```python
from build123d import *

# Parameters (mm, degrees)
ESTRUSIONE_ESTRUSIONE1_DEPTH      = 48
ESTRUSIONE_ESTRUSIONE1_DEPTH_BACK = 5
SCHIZZO2_W                        = 45
SCHIZZO2_H                        = 3
ESTRUSIONE_ESTRUSIONE2_DEPTH      = 5
CORPO_SPOSTA_COPIA1_START         = 131.104025403
CORPO_SPOSTA_COPIA1_OUTLINE_W     = 3
CORPO_SPOSTA_COPIA1_OUTLINE_H     = 43
CORPO_SPOSTA_COPIA1_DEPTH         = 31.786555516
CORPO_SPOSTA_COPIA1_2_OUTLINE_W   = 3
CORPO_SPOSTA_COPIA1_2_OUTLINE_H   = 5
CORPO_SPOSTA_COPIA1_2_DEPTH       = 5
CORPO_SPOSTA_COPIA1_START_2       = 157.890580919
CORPO_SPOSTA_COPIA1_3_OUTLINE_W   = 3
CORPO_SPOSTA_COPIA1_3_OUTLINE_H   = 5
CORPO_SPOSTA_COPIA1_3_DEPTH       = 5
CORPO_SPOSTA_COPIA1_4_OUTLINE_W   = 3
CORPO_SPOSTA_COPIA1_4_OUTLINE_H   = 45
CORPO_SPOSTA_COPIA1_4_DEPTH       = 31.786555516
CORPO_SPOSTA_COPIA1_START_3       = 136.104025403
CORPO_SPOSTA_COPIA1_5_OUTLINE_W   = 3
CORPO_SPOSTA_COPIA1_5_OUTLINE_H   = 3
CORPO_SPOSTA_COPIA1_5_DEPTH       = 21.786555516


# Read off the part's stored shape, not the designer's step: Corpo-Sposta/copia1
with BuildPart() as part:
    # Schizzo1 → Estrusione-Estrusione1 (new, two sides: drawn at the far end of the back side and taken through both)
    with BuildSketch(Plane.XY.offset(-ESTRUSIONE_ESTRUSIONE1_DEPTH_BACK)):
        Polygon((198.017140331, -69.250735791), (177.803209237, -77.377911869), (178.92231814, -80.161362114), (199.136249234, -72.034186035), align=None)
    extrude(amount=ESTRUSIONE_ESTRUSIONE1_DEPTH + ESTRUSIONE_ESTRUSIONE1_DEPTH_BACK)

    # Schizzo2 → Estrusione-Estrusione2 (add)
    with BuildSketch(Plane(origin=(146.49352536, 58.898918246, 0), x_dir=(0, 0, -1), z_dir=(0.9278167482016688, 0.3730363008562049, 0))):
        with Locations((-22.5, -139.619574027)):
            Rectangle(SCHIZZO2_W, SCHIZZO2_H)
    estrusione_estrusione2 = extrude(amount=ESTRUSIONE_ESTRUSIONE2_DEPTH)

    # Specchia1: Estrusione-Estrusione2 across plane
    add(estrusione_estrusione2.mirror(Plane(origin=(136.386559813, 54.835330207, 0), x_dir=(0, 0, 1), z_dir=(0.9278167482016688, 0.37303630085620504, 0))))

    # Corpo-Sposta/copia1 outline → Corpo-Sposta/copia1 (cut)
    with BuildSketch(Plane(origin=(0, 0, 0), x_dir=(-0.373036300856202, 0.92781674820167, 0), z_dir=(0.92781674820167, 0.373036300856202, 0)).offset(CORPO_SPOSTA_COPIA1_START)):
        with Locations((-139.619574027, 26.5)):
            Rectangle(CORPO_SPOSTA_COPIA1_OUTLINE_W, CORPO_SPOSTA_COPIA1_OUTLINE_H)
    extrude(amount=CORPO_SPOSTA_COPIA1_DEPTH, mode=Mode.SUBTRACT)

    # Corpo-Sposta_copia1 2 outline → Corpo-Sposta_copia1 2 (cut)
    with BuildSketch(Plane(origin=(0, 0, 0), x_dir=(-0.373036300856202, 0.92781674820167, 0), z_dir=(0.92781674820167, 0.373036300856202, 0)).offset(CORPO_SPOSTA_COPIA1_START)):
        with Locations((-139.619574027, 2.5)):
            Rectangle(CORPO_SPOSTA_COPIA1_2_OUTLINE_W, CORPO_SPOSTA_COPIA1_2_OUTLINE_H)
    extrude(amount=CORPO_SPOSTA_COPIA1_2_DEPTH, mode=Mode.SUBTRACT)

    # Corpo-Sposta_copia1 3 outline → Corpo-Sposta_copia1 3 (cut)
    with BuildSketch(Plane(origin=(0, 0, 0), x_dir=(-0.373036300856202, 0.92781674820167, 0), z_dir=(0.92781674820167, 0.373036300856202, 0)).offset(CORPO_SPOSTA_COPIA1_START_2)):
        with Locations((-139.619574027, 2.5)):
            Rectangle(CORPO_SPOSTA_COPIA1_3_OUTLINE_W, CORPO_SPOSTA_COPIA1_3_OUTLINE_H)
    extrude(amount=CORPO_SPOSTA_COPIA1_3_DEPTH, mode=Mode.SUBTRACT)

    # Corpo-Sposta_copia1 4 outline → Corpo-Sposta_copia1 4 (add)
    with BuildSketch(Plane(origin=(0, 0, 0), x_dir=(-0.373036300856202, 0.92781674820167, 0), z_dir=(0.92781674820167, 0.373036300856202, 0)).offset(CORPO_SPOSTA_COPIA1_START)):
        with Locations((-139.619574027, -22.5)):
            Rectangle(CORPO_SPOSTA_COPIA1_4_OUTLINE_W, CORPO_SPOSTA_COPIA1_4_OUTLINE_H)
    extrude(amount=CORPO_SPOSTA_COPIA1_4_DEPTH)

    # Corpo-Sposta_copia1 5 outline → Corpo-Sposta_copia1 5 (add)
    with BuildSketch(Plane(origin=(0, 0, 0), x_dir=(-0.373036300856202, 0.92781674820167, 0), z_dir=(0.92781674820167, 0.373036300856202, 0)).offset(CORPO_SPOSTA_COPIA1_START_3)):
        with Locations((-139.619574027, -46.5)):
            Rectangle(CORPO_SPOSTA_COPIA1_5_OUTLINE_W, CORPO_SPOSTA_COPIA1_5_OUTLINE_H)
    extrude(amount=CORPO_SPOSTA_COPIA1_5_DEPTH)


solid = part.part
```
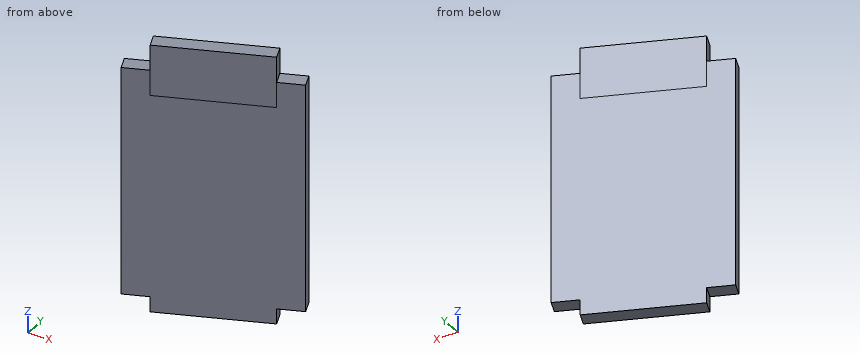
The model under review builds one solid part; all positions refer to its coordinate system, in mm. Round coordinates to 2 decimals unless told otherwise and drop trailing zeros. Order: outer loops, then holes, each group sorted by start corner. A loop starts at its lowest first (then second) coordinate and runs counter-clockwise, first axis right, second up. Notation, with made-up numbers: (65, 82.25) -> (93, 82.25) arc R31 ccw to (93, 116.25) -> close; hole circle Ø7 at (1, -22.5). An arc over 180 degrees is marked (long way). One line per item, written item: value. Start each with the question number.
Q1. Take a section at A-A (y = -70.75). Write out the cut boundary in (x, z).
Q2. Take a section at B-B (z = -44). Write out the cut boundary in (x, y).
Q3. Take a section at C-C (x = 191). Write out the cut boundary in (y, z), and give its area (3 significant figures).
Q4. Clearance check with flat-ended pins moving along their axes: pin 1 Ø2.5 at (x, y) = (177, -80.5) entering from +Z; pin 2 Ø6 at (x, y) = (198, -75) entering from +Z; pin 3 Ø5 at (x, z) = (197.5, -7) entering from +Y; pin 4 Ø3 at (y, z) = (-69.5, -31.5) entering from -X. State where each tip first meets the part, or that it passes through.
Q5. Take a section at D-D (y = -73). Write out the cut boundary in (x, z), and give its area (3 significant figures).
Q6. Wall thickness on line 1 (Z direction, x = 200.5, y = -70.5); line 2 (X direction, y = -73.25, z = -42.5); line 3 (X direction, y = -70.75, z = -21): over which ranges is each line inside the solid? List them lowest first.
Reported:
1. outline: (194.29, -48) -> (198.62, -48) -> (198.62, -45) -> (202.33, -45) -> (202.33, 0) -> (198.62, 0) -> (198.62, 5) -> (194.29, 5) -> close
2. outline: (173.16, -79.24) -> (174.28, -82.03) -> (203.78, -70.17) -> (202.66, -67.39) -> close
3. outline: (-75.31, -48) -> (-72.07, -48) -> (-72.07, 5) -> (-75.31, 5) -> close
3. area: 171 mm2
4. pin 1: stops at z = 0
4. pin 2: stops at z = 5
4. pin 3: stops at y = -68.45
4. pin 4: stops at x = 193.67
5. outline: (188.69, -48) -> (196.73, -48) -> (196.73, 5) -> (188.69, 5) -> close
5. area: 426 mm2
6. line 1: z = -45 to 0
6. line 2: x = 188.07 to 196.11
6. line 3: x = 194.29 to 202.33
